Verification items for this drawing (mm, ordinates from the low corner). Round coordinates to 2 decimals unless told otherwise and drop trailing zeros. Write each loop counter-clockwise with the first axis right and the second up, starting at its lowest first coordinate (ties: lowest second). Pieces come first, ordered by that corner, then holes.
Item 1: Scan lines: probe 1 along X at (y, z) = (57.15, 6.75); probe 2 along Y at (x, z) = (68.9, 7). Record each from-to range of solid material in increasing order.
Item 2: Cross-section at A-A (x = 53.9). Enter the section's corners in (y, z), then the cut area to 3 significant figures.
Item 3: Cross-section at B-B (y = 57.15). Enter the section's corners in (x, z), then the cut area to 3 significant figures.
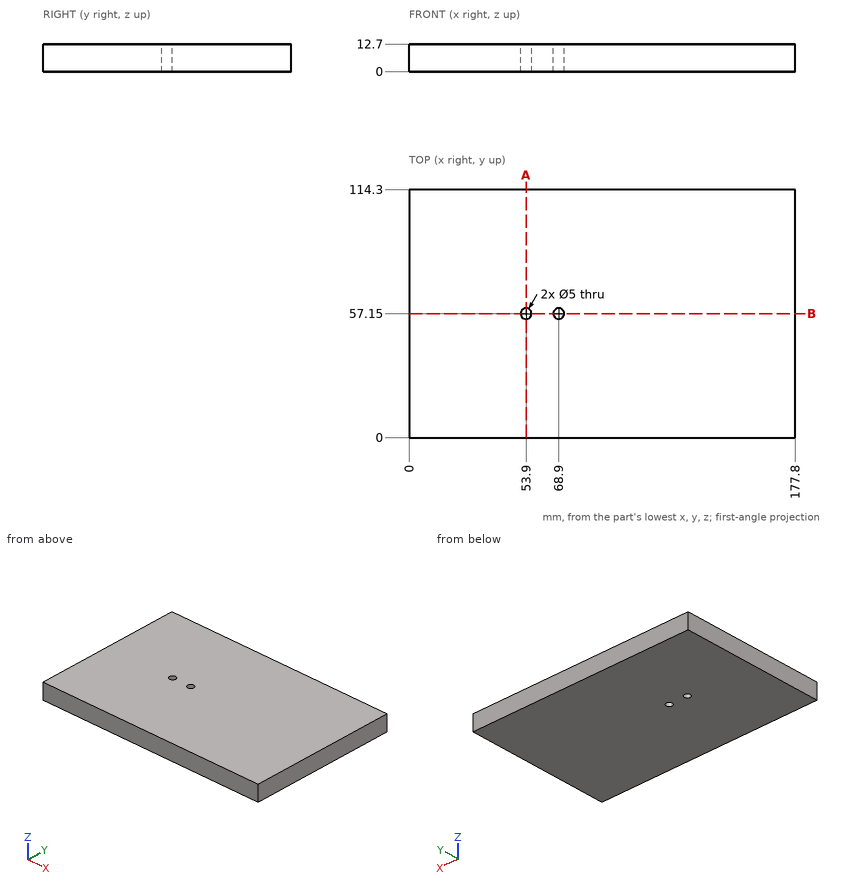
Resolved:
1. probe 1: x = 0 to 51.4, 56.4 to 66.4, 71.4 to 177.8
1. probe 2: y = 0 to 54.65, 59.65 to 114.3
2. outline: (0, 0) - (54.65, 0) - (54.65, 12.7) - (0, 12.7) - close; (59.65, 0) - (114.3, 0) - (114.3, 12.7) - (59.65, 12.7) - close
2. area: 1,390 mm2
3. outline: (0, 0) - (51.4, 0) - (51.4, 12.7) - (0, 12.7) - close; (56.4, 0) - (66.4, 0) - (66.4, 12.7) - (56.4, 12.7) - close; (71.4, 0) - (177.8, 0) - (177.8, 12.7) - (71.4, 12.7) - close
3. area: 2,130 mm2
